```python
from build123d import *

# Parameters (mm, degrees)
F1_DEPTH        = 2
F3_R            = 1.5
F6_DEPTH        = 12.5
F5_R            = 1.5
F7_DEPTH        = 12.5
F8_R            = 1.25
F9_DEPTH        = 40
F11_D           = 4.4
F11_DEPTH       = 14.1
F11_CSINK_D     = 8.96
F11_CSINK_ANGLE = 90
F11_TIP         = 1.3218933619


with BuildPart() as f1:
    # F0 (on Top) → F1 (new body)
    with BuildSketch(Plane.XY):
        with BuildLine():
            ThreePointArc((20, 5), (18.5355339059, 8.5355339059), (15, 10))
            Line((15, 10), (-15, 10))
            ThreePointArc((-15, 10), (-18.5355339059, 8.5355339059), (-20, 5))
            Line((-20, 5), (-20, -10))
            Line((-20, -10), (20, -10))
            Line((20, -10), (20, 5))
        make_face()
    extrude(amount=F1_DEPTH)

    # F3 (on offset) → F6 (join, through all)
    with BuildSketch(Plane.YZ.offset(7.5)):
        with Locations((-10, 3.25)):
            Circle(F3_R)
    extrude(amount=F6_DEPTH)

    # F5 (on offset) → F7 (join, through all)
    with BuildSketch(Plane.YZ.offset(-7.5)):
        with Locations((-10, 3.25)):
            Circle(F5_R)
    extrude(amount=-F7_DEPTH)

    # F8 (on face) → F9 (cut, through all)
    with BuildSketch(Plane.YZ.offset(20)):
        with Locations((-10, 3.25)):
            Circle(F8_R)
    extrude(amount=-F9_DEPTH, mode=Mode.SUBTRACT)

    # F11
    with Locations(Plane.XY.offset(2)):
        with Locations((-12.5, 0), (12.5, 0)):
            CounterSinkHole(F11_D / 2, F11_CSINK_D / 2, depth=F11_DEPTH, counter_sink_angle=F11_CSINK_ANGLE)
            with Locations((0, 0, -(F11_DEPTH + F11_TIP / 2))):  # 118° drill point
                Cone(0, F11_D / 2, F11_TIP, mode=Mode.SUBTRACT)


solid = f1.part
```
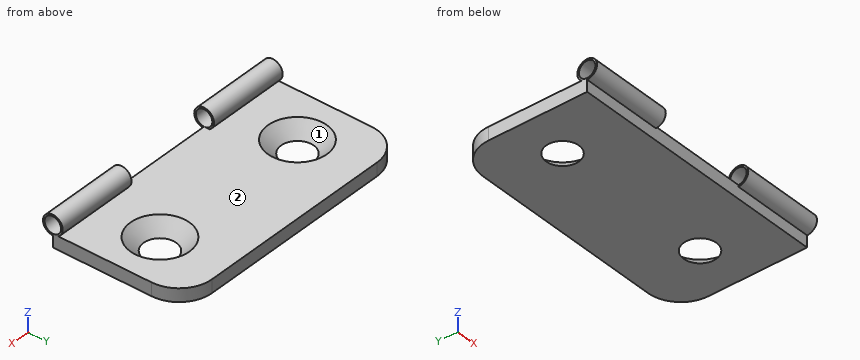
Model file for the job. Use its own axes, mm. Face numbers are marked on the shaded views. Coordinates: 2 decimals unless noted, no trailing zeros. Order: outer loops, then holes, each group sorted by start corner. A loop starts at its lowest first (then second) coordinate and runs counter-clockwise, first axis right, second up. Notation, with made-up numbers: M -30.5,-34.75 L 6.5,-34.75 A31 cw 6.5,2.25 Z; hole C 51.5,-2 d2. An arc over 180 degrees is marked long. Answer as CSV lines item,"result".
(1) Flat gauge pins, fed straight in: pin 1 (10 mm diameter, centred on x = 11, y = 0.5, fed in from +Z); pin 2 (0.9 mm diameter, centred on y = -10, z = 4, fed in from -X). Where does each tip first touch, or does it go through?
Geometry says:
pin 1,"stops at z = 2"
pin 2,"passes through"
(2) Band-saw the part on D-D, the plane x = -5. List the corners of the cut face in (y, z), then the cut area to 3 significant figures.
Geometry says:
outline,"M -10,0 L 10,0 L 10,2 L -10,2 Z"
area,"40.0 mm2"
(3) Band-saw the part on C-C, the plane x = 12.5. List the corners of the cut face in (y, z).
Geometry says:
outline,"M -10,0 L -2.48,0 L -4.48,2 L -9.17,2 A1.5 ccw long -10,1.75 Z; M 2.48,0 L 10,0 L 10,2 L 4.48,2 Z; hole C -10,3.25 d2.5"
(4) Band-saw the part on A-A, the plane y = 0. List the corners of the cut face in (x, z), then the cut area to 3 significant figures.
Geometry says:
outline,"M -20,0 L -14.98,0 L -16.98,2 L -20,2 Z; M -10.02,0 L 10.02,0 L 8.02,2 L -8.02,2 Z; M 14.98,0 L 20,0 L 20,2 L 16.98,2 Z"
area,"52.2 mm2"
(5) Wall check: line 1 along Y through (x, z) = (-11, 3.3); line 2 along Z through (x, y) = (-4.5, -3); line 3 along X through (y, z) = (0.5, 1.5). Give the ranges that are in metal, low to high.
Geometry says:
line 1,"y = -11.5 to -11.25, -8.75 to -8.5"
line 2,"z = 0 to 2"
line 3,"x = -20 to -16.45, -8.55 to 8.55, 16.45 to 20"
(6) Band-saw the part on B-B, the plane z = 1.05. List the corners of the cut face in (x, y).
Geometry says:
outline,"M -20,-10 L 20,-10 L 20,5 A5 ccw 15,10 L -15,10 A5 ccw -20,5 Z; hole C -12.5,0 d7.06; hole C 12.5,0 d7.06"
(7) Pull direction Y, two halves, no side cores. Call the marked faces 1 and 2: +Y half, -Y half, draft (parallel to the pull), parting line (faces both ways), or undercut.
Geometry says:
face 1,"undercut"
face 2,"draft"
